```python
from build123d import *

# Parameters (mm, degrees)
SKETCH_R        = 25
PAD_DEPTH       = 25
PAD_TAPER       = 15
SKETCH001_R     = 19.440567
POCKET_DEPTH    = 20
POCKET_TAPER    = 15
SKETCH002_R     = 10
PAD001_DEPTH    = 25
PAD001_TAPER    = 15
SKETCH003_R     = 2.074758
POCKET001_DEPTH = 17


with BuildPart() as part:
    # Sketch → Pad (new body)
    with BuildSketch(Plane.XY):
        Circle(SKETCH_R)
    extrude(amount=PAD_DEPTH, taper=PAD_TAPER)

    # Sketch001 (on Face2 of Pad) → Pocket (cut)
    with BuildSketch(Plane(origin=(0, 0, 0), x_dir=(1, 0, 0), z_dir=(0, 0, -1))):
        Circle(SKETCH001_R)
    extrude(amount=-POCKET_DEPTH, taper=POCKET_TAPER, mode=Mode.SUBTRACT)

    # Sketch002 (on Face5 of Pocket) → Pad001 (join)
    with BuildSketch(Plane(origin=(0, 0, 20), x_dir=(1, 0, 0), z_dir=(0, 0, -1))):
        Circle(SKETCH002_R)
    extrude(amount=PAD001_DEPTH, taper=PAD001_TAPER)

    # Sketch003 (on Face7 of Pad001) → Pocket001 (cut)
    with BuildSketch(Plane(origin=(0, 0, -5), x_dir=(1, 0, 0), z_dir=(0, 0, -1))):
        Circle(SKETCH003_R)
    extrude(amount=-POCKET001_DEPTH, mode=Mode.SUBTRACT)


solid = part.part
```
Design review of the part built by this model. Coordinates are the model's own, in mm. A direction names the side the tool comes from. Give positions to 0.01 mm unless a question says otherwise; leave off trailing zeros. Order: outer loops, then holes, each group sorted by start corner. A loop starts at its lowest first (then second) coordinate and runs counter-clockwise, first axis right, second up. Notation, with made-up numbers: (2.25, -17) - (47.25, -17) arc R31 ccw to (47.25, 11) - close; hole circle Ø2 at (39.5, -4.5). An arc over 180 degrees is marked (long way). Use a Markdown table: item, result. Add a question column.
(1) Machinability: for faces 5 (the face through (0, 0, 25)), 6 (the face through (0, 0, 12)), which of the approach directions +Z, -Z, +X, -X, +Y, -Y give a long, thin tool a straight path to every point of the face, cutting with its end or side? Answer none if there is none.
(2) Add section A-A on x = 0. Give the boundary of the cut face in (y, z).
(3) Add section B-B on z = -1.5. Give the boundary of the cut face in (x, y), then the cut area to 3 significant figures.
(4) Mouldability with a two-part tool opening along X and no side actions: class faces 1 (the face through (9.282, -17.846, 18.231)), 2 (the face through (7.17, 13.78, 14.58)), 3 (the face through (-4.65, 3.565, 4.547)), 4 (the face through (-2, 1, -5)) as +X half, -X half, draft (parallel to the pull), parting line (faces both ways), or undercut.
(5) Wall thickness on probe 1 along Y at (x, z) = (0, 1); probe 2 along Y at (x, z) = (0, 7); probe 3 along Y at (x, z) = (6.5, 18): over which ranges is each line inside the solid? List them lowest first. Write a range as [from, to].
(6) Clearance check with flat-ended pins moving along their axes: P1, Ø1, axis at y = 2.5, z = 15.5, coming from the -X side; P2, Ø1.5, axis at x = -18, y = -13.5, coming from the -Z side; P3, Ø10, axis at x = 5.5, z = 14.5, coming from the +Y side. State where each tip first meets the part, or that it passes through.
Report:
| question | item | result |
|---|---|---|
| 1 | face 5 | +Z, +X, -X, +Y, -Y |
| 1 | face 6 | -Z |
| 2 | outline | (-25, 0) - (-19.44, 0) - (-14.08, 20) - (-10, 20) - (-3.3, -5) - (-2.07, -5) - (-2.07, 12) - (2.07, 12) - (2.07, -5) - (3.3, -5) - (10, 20) - (14.08, 20) - (19.44, 0) - (25, 0) - (18.3, 25) - (-18.3, 25) - close |
| 3 | outline | circle Ø8.48 at (0, 0); hole circle Ø4.15 at (0, 0) |
| 3 | area | 42.9 mm² |
| 4 | face 1 | parting line |
| 4 | face 2 | undercut |
| 4 | face 3 | undercut |
| 4 | face 4 | draft |
| 5 | probe 1 | y = [-24.73, -19.17], [-4.91, -2.07], [2.07, 4.91], [19.17, 24.73] |
| 5 | probe 2 | y = [-23.12, -17.56], [-6.52, -2.07], [2.07, 6.52], [17.56, 23.12] |
| 5 | probe 3 | y = [-19.1, -13.09], [-6.88, 6.88], [13.09, 19.1] |
| 6 | P1 | stops at x = -20.84 |
| 6 | P2 | stops at z = 0 |
| 6 | P3 | stops at y = 22.07 |
